Model file for the job. Use its own axes, mm. Face numbers are marked on the shaded views. A direction names the side the tool comes from. Round coordinates to 2 decimals unless told otherwise and drop trailing zeros. Write each loop counter-clockwise with the first axis right and the second up, starting at its lowest first coordinate (ties: lowest second). Pieces come first, ordered by that corner, then holes.
Autodesk Inventor part; units mm, degrees
ref_plane "YZ Plane" through (0, 0, 0) normal (1, 0, 0) x (0, 1, 0)
ref_plane "XZ Plane" through (0, 0, 0) normal (0, 1, 0) x (-1, 0, 0)
ref_plane "XY Plane" through (0, 0, 0) normal (0, 0, 1) x (1, 0, 0)
sketch "Head Revolution Profile" plane through (0, 0, 0) normal (0, 0, 1) x (1, 0, 0)
  line L0 (0, -5) -> (5, 0)
  line L1 (5, 0) -> (0, 0)
  line L2 (0, 0) -> (0, -5)
  dimension "d0" = 0
  dimension "d1" = 45
  dimension "d2" = 5
  dimension "d3" = 0
revolve "Head" add sketch "Head Revolution Profile" angle 360 about axis through (0, 0, 0) along (0, -1, 0)
sketch "Body Cross Section" plane through (0, 0, 0) normal (0, 1, 0) x (1, 0, 0)
  circle A0 centre (0, 0) radius 2.5
  point P0 (0, 0)
  dimension "d5" = 5
extrude "Body" add sketch "Body Cross Section" against normal blind 18
thread "Thread"
sketch "Key Socket Cutout Outline" plane through (0, 0, 0) normal (0, 1, 0) x (1, 0, 0)
  line L0 (0.866, 1.5) -> (1.7321, 0)
  line L1 (1.7321, 0) -> (0.866, -1.5)
  line L2 (0.866, -1.5) -> (-0.866, -1.5)
  line L3 (-0.866, -1.5) -> (-1.7321, 0)
  line L4 (-1.7321, 0) -> (-0.866, 1.5)
  line L5 (-0.866, 1.5) -> (0.866, 1.5)
  point P0 (0, 0)
  point P1 (0, 0)
  dimension "d10" = 3
extrude "Key Socket Cutout" cut sketch "Key Socket Cutout Outline" against normal blind 2.3
properties part number "SSK-M5-18-A4" material "Stainless Steel AISI 317"
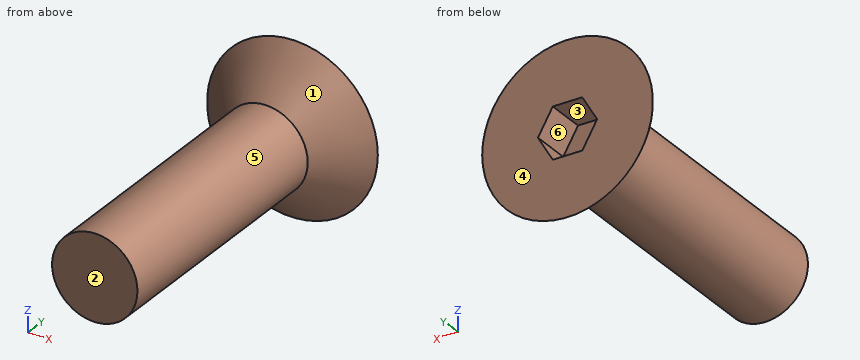
1) Cut at A-A on y = -1.5. List the corners of the cut face in (x, z).
2) Flat gauge pins, fed straight in: pin 1 Ø6 at (x, y) = (-1, -6) entering from +Z; pin 2 Ø3 at (y, z) = (-11.5, -0.5) entering from +X; pin 3 Ø0.5 at (x, y) = (-0.5, -1.5) entering from -Z. Where does each tip first touch, or does it go through?
3) Cut at C-C on y = -7.75. List the corners of the cut face in (x, z), and give its area (3 significant figures).
4) Pull direction X, two halves, no side cores. Call the marked faces 1, 2 and 3: released by +X, released by -X, zero draft, split by the parting line, or undercut.
5) Wall check: probe 1 along X at (y, z) = (-11, 0); probe 2 along X at (y, z) = (-13.75, -2). Give the ranges that are in metal, low to high.
6) Cut at B-B on x = 0. List the corners of the cut face in (y, z).
7) Which spindle directions (+Z, -Z, +X, -X, +Y, -Y) get a long thin tool onto all of the face, cutting with end or side? Do the marked faces 4, 5 and 6. Say none if no direction does.
Result sheet:
1. outline: circle Ø7 at (0, 0); hole (-1.73, 0) - (-0.87, -1.5) - (0.87, -1.5) - (1.73, 0) - (0.87, 1.5) - (-0.87, 1.5) - close
2. pin 1: stops at z = 2.5
2. pin 2: stops at x = 2.5
2. pin 3: stops at z = -3.72
3. outline: circle Ø5 at (0, 0)
3. area: 19.6 mm2
4. face 1: split by the parting line
4. face 2: zero draft
4. face 3: undercut
5. probe 1: x = -2.5 to 2.5
5. probe 2: x = -1.5 to 1.5
6. outline: (-18, -2.5) - (-2.5, -2.5) - (0, -5) - (0, -1.5) - (-2.3, -1.5) - (-2.3, 1.5) - (0, 1.5) - (0, 5) - (-2.5, 2.5) - (-18, 2.5) - close
7. face 4: +Z, -Z, +X, -X, +Y
7. face 5: -Y
7. face 6: +Y
